```python
from build123d import *

# Parameters (mm, degrees)
SKETCH4_W           = 14.1
SKETCH4_H           = 64
BOSS_EXTRUDE1_DEPTH = 16.3
FILLET1_R           = 1.5
SKETCH5_W           = 11.6
SKETCH5_H           = 24.3
CUT_EXTRUDE1_DEPTH  = 16.3
SKETCH6_W           = 4.05
SKETCH6_H           = 4.2
CUT_EXTRUDE2_DEPTH  = 12.7
FILLET2_R           = 1
SKETCH7_R           = 1
CUT_EXTRUDE3_DEPTH  = 16.3


with BuildPart() as part:
    # Sketch4 → Boss-Extrude1 (new body)
    with BuildSketch(Plane.XY.offset(30)):
        with Locations((-182.786990356, 243.547210693)):
            Rectangle(SKETCH4_W, SKETCH4_H)
    extrude(amount=BOSS_EXTRUDE1_DEPTH)

    # Fillet1
    fillet1_edges = [part.edges().sort_by_distance(p)[0] for p in [
        (-189.836990356, 275.547210693, 38.15),
        (-175.736990356, 275.547210693, 38.15),
        (-175.736990356, 211.547210693, 38.15),
        (-189.836990356, 211.547210693, 38.15),
    ]]
    fillet(fillet1_edges, radius=FILLET1_R)

    # Sketch5 → Cut-Extrude1 (cut)
    with BuildSketch(Plane.XY.offset(46.3)):
        with Locations((-182.736990356, 259.597210693)):
            Rectangle(SKETCH5_W, SKETCH5_H)
        with Locations((-182.736990356, 227.497210693)):
            Rectangle(SKETCH5_W, SKETCH5_H)
    extrude(amount=-CUT_EXTRUDE1_DEPTH, mode=Mode.SUBTRACT)

    # Sketch6 → Cut-Extrude2 (cut)
    with BuildSketch(Plane.XY.offset(46.3)):
        with Locations((-187.811990356, 243.547210693)):
            Rectangle(SKETCH6_W, SKETCH6_H)
        with Locations((-177.761990356, 243.547210693)):
            Rectangle(SKETCH6_W, SKETCH6_H)
    extrude(amount=-CUT_EXTRUDE2_DEPTH, mode=Mode.SUBTRACT)

    # Fillet2
    fillet2_edges = [part.edges().sort_by_distance(p)[0] for p in [
        (-189.836990356, 241.447210693, 39.95),
        (-189.836990356, 245.647210693, 39.95),
        (-175.736990356, 245.647210693, 39.95),
        (-175.736990356, 241.447210693, 39.95),
    ]]
    fillet(fillet2_edges, radius=FILLET2_R)

    # Sketch7 → Cut-Extrude3 (cut)
    with BuildSketch(Plane.XY.offset(46.3)):
        with Locations((-183.086103711, 273.651926582)):
            Circle(SKETCH7_R)
        with Locations((-183.086103711, 213.475534384)):
            Circle(SKETCH7_R)
        with Locations((-183.098908316, 246.016003292)):
            Circle(SKETCH7_R)
        with Locations((-183.18196106, 241.016693115)):
            Circle(SKETCH7_R)
    extrude(amount=-CUT_EXTRUDE3_DEPTH, mode=Mode.SUBTRACT)


solid = part.part
```
The model under review builds one solid part; all positions refer to its coordinate system, in mm. A direction names the side the tool comes from. Round coordinates to 2 decimals unless told otherwise and drop trailing zeros. Loops run counter-clockwise (first coordinate to the right, second up) from the corner with the lowest first, then second, coordinate; pieces in that order, holes last. Notation, with made-up numbers: M 88.5,-2.75 L 123.5,-2.75 A25 ccw 123.5,11.25 Z; hole C 38.5,-36 d9. An arc over 180 degrees is marked long. Write item = value, one per line.
Item 1: Take a section at A-A on x = -185. Write out the cut boundary in (y, z).
Return value:
outline = M 211.55,30 L 215.35,30 L 215.35,46.3 L 211.55,46.3 Z; M 239.65,30 L 247.45,30 L 247.45,46.3 L 239.65,46.3 Z; M 271.75,30 L 275.55,30 L 275.55,46.3 L 271.75,46.3 Z
Item 2: Insertion check: P1, Ø3, axis at x = -177, y = 243, coming from the +Z side; P2, Ø1.3, axis at y = 243.5, z = 37.5, coming from the -X side; P3, Ø1.2, axis at x = -183.09, y = 273.65, coming from the +Z side; P4, Ø3, axis at x = -180, y = 247.5, coming from the +Z side. Each pin has a flat end and moves straight along its axis. Give the tip position at first contact, or say it passes through.
Return value:
P1 = 33.6
P2 = -185.79
P3 = through
P4 = 46.3
Item 3: Take a section at C-C on z = 31.75. Write out the cut boundary in (x, y), then the cut area to 3 significant figures.
Return value:
outline = M -189.84,213.05 A1.5 ccw -188.34,211.55 L -177.24,211.55 A1.5 ccw -175.74,213.05 L -175.74,274.05 A1.5 ccw -177.24,275.55 L -188.34,275.55 A1.5 ccw -189.84,274.05 Z; hole M -188.54,215.35 L -176.94,215.35 L -176.94,239.65 L -188.54,239.65 Z; hole M -188.54,247.45 L -176.94,247.45 L -176.94,271.75 L -188.54,271.75 Z; hole C -183.18,241.02 d2; hole C -183.1,246.02 d2; hole C -183.09,213.48 d2; hole C -183.09,273.65 d2
area = 324 mm2
Item 4: Take a section at D-D on z = 34.5. State how many separate pieces and enclosed holes the cut face has, then the cut area to 3 significant figures.
Return value:
separate_pieces = 1
enclosed_holes = 6
area = 289 mm2
Item 5: The part is to be moulded in two halves that separate along Y. For faces 1 (the flat face through (-183, 211.547, 38)), 2 (the flat face through (-187, 241.447, 40)), 3 (the flat face through (-175.737, 243, 33)), 4 (the flat face through (-183, 275.547, 38)), say which applies: released by +Y, released by -Y, zero draft, split by the parting line, or undercut.
Return value:
face_1 = released by -Y
face_2 = undercut
face_3 = zero draft
face_4 = released by +Y
Item 6: For line 1 (Y direction, x = -179.5, z = 31.25); line 2 (Y direction, x = -187.75, z = 41); line 3 (X direction, y = 265, z = 38), list the stretches that pass through material, from the lowest coordinate up. Write a range as [from, to].
Return value:
line_1 = [211.55, 215.35], [239.65, 247.45], [271.75, 275.55]
line_2 = [211.55, 215.35], [239.65, 241.45], [245.65, 247.45], [271.75, 275.55]
line_3 = [-189.84, -188.54], [-176.94, -175.74]
Item 7: Take a section at B-B on y = 237. Write out the cut boundary in (x, z).
Return value:
outline = M -189.84,30 L -188.54,30 L -188.54,46.3 L -189.84,46.3 Z; M -176.94,30 L -175.74,30 L -175.74,46.3 L -176.94,46.3 Z
Item 8: Machinability: for faces 5 (the flat face through (-176.937, 227, 38)), 6 (the cylindrical face through (-176.188, 211.975, 38.264)), 7 (the flat face through (-178, 245.647, 40)), 8 (the flat face through (-185.787, 244, 40)), 9 (the cylindrical face through (-176.165, 275.096, 38.264)), which of the approach directions +Z, -Z, +X, -X, +Y, -Y give a long, thin tool a straight path to every point of the face, cutting with its end or side? Answer none if there is none.
Return value:
face_5 = +Z, -Z
face_6 = +Z, -Z, +X, -Y
face_7 = +Z, +X
face_8 = +Z, -X
face_9 = +Z, -Z, +X, +Y
